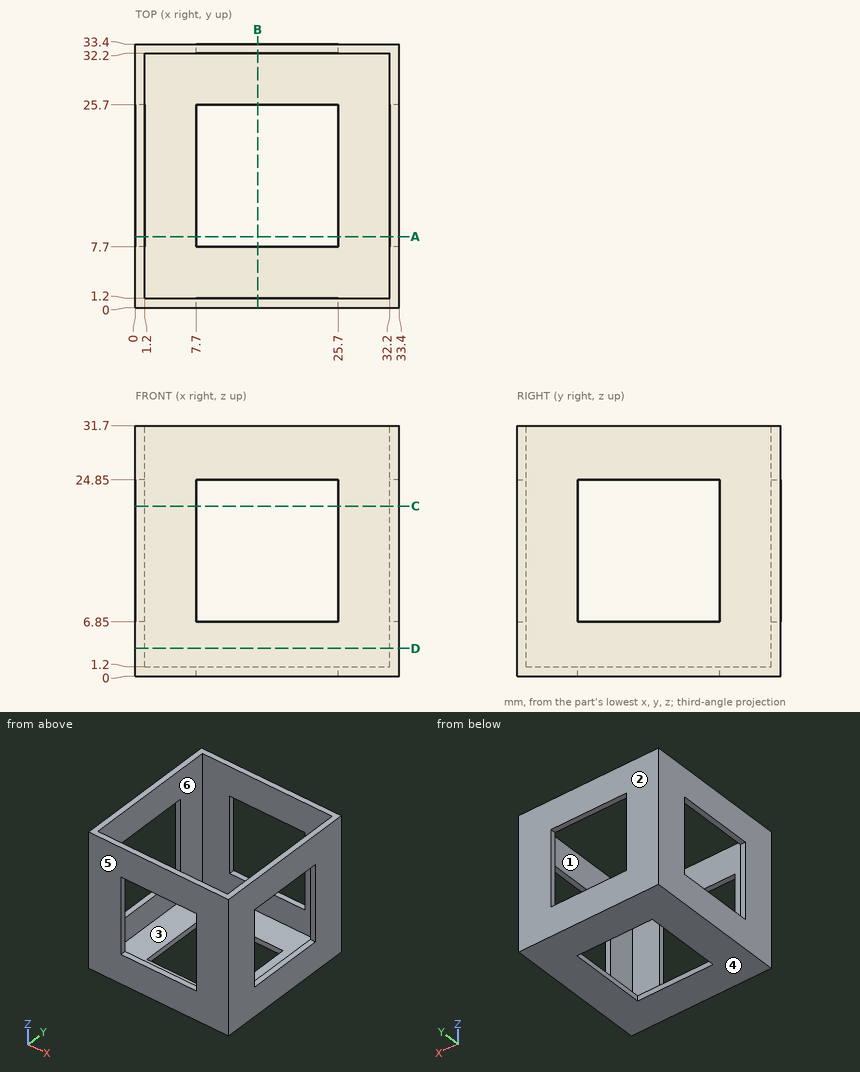
Design review of the part shown in the three views and the two pictorial views. Dimensions are in mm from the part's minimum x, y and z. A direction names the side the tool comes from. Round coordinates to 2 decimals unless told otherwise and drop trailing zeros. Order: outer loops, then holes, each group sorted by start corner. A loop starts at its lowest first (then second) coordinate and runs counter-clockwise, first axis right, second up. Notation, with made-up numbers: (-29, -23.5) -> (17, -23.5) arc R23 cw to (17, 12.5) -> close; hole circle Ø8 at (89, 31). An arc over 180 degrees is marked (long way). Write item = value, one per line. Start each with the question number.
1) Insertion check: pin 1 (3 mm diameter, centred on x = 15, z = 8, fed in from -Y); pin 2 (12 mm diameter, centred on x = 23.5, y = 21, fed in from +Z). Each pin has a flat end and moves straight along its axis. Give the tip position at first contact, or say it passes through.
2) Tool access review of the marked faces 5 and 6: name each direction out of +Z, -Z, +X, -X, +Y, -Y from which nothing blocks a thin tool from reaching the whole face with its end or side.
3) Take a section at A-A on y = 9. State the section outline as (x, z) points.
4) Take a section at D-D on z = 3.5. State the section outline as (x, y) points, plus the area to 3 significant figures.
5) To check wall thickness, follow line 1 (X direction, y = 15.5, z = 27); line 2 (Y direction, x = 18, z = 1). State the ranges of each line that lie inside material, in increasing order. Write a range as from..to.
6) Take a section at C-C on z = 21.5. State the section outline as (x, y) points, plus the area to 3 significant figures.
7) The part is to be moulded in two halves that separate along Y. For the marked faces 1, 2, 3 and 4, say which applies: +Y half, -Y half, draft (parallel to the pull), parting line (faces both ways), or undercut.
Verdict:
q1.pin_1 = 0
q1.pin_2 = 1.2
q2.face_5 = +Z, -Z, +X, -X, -Y
q2.face_6 = +Z
q3.outline = (0, 0) -> (7.7, 0) -> (7.7, 1.2) -> (1.2, 1.2) -> (1.2, 6.85) -> (0, 6.85) -> close; (0, 24.85) -> (1.2, 24.85) -> (1.2, 31.7) -> (0, 31.7) -> close; (25.7, 0) -> (33.4, 0) -> (33.4, 6.85) -> (32.2, 6.85) -> (32.2, 1.2) -> (25.7, 1.2) -> close; (32.2, 24.85) -> (33.4, 24.85) -> (33.4, 31.7) -> (32.2, 31.7) -> close
q4.outline = (0, 0) -> (33.4, 0) -> (33.4, 33.4) -> (0, 33.4) -> close; hole (1.2, 1.2) -> (32.2, 1.2) -> (32.2, 32.2) -> (1.2, 32.2) -> close
q4.area = 155 mm2
q5.line_1 = 0..1.2, 32.2..33.4
q5.line_2 = 0..7.7, 25.7..33.4
q6.outline = (0, 0) -> (7.7, 0) -> (7.7, 1.2) -> (1.2, 1.2) -> (1.2, 7.7) -> (0, 7.7) -> close; (0, 25.7) -> (1.2, 25.7) -> (1.2, 32.2) -> (7.7, 32.2) -> (7.7, 33.4) -> (0, 33.4) -> close; (25.7, 0) -> (33.4, 0) -> (33.4, 7.7) -> (32.2, 7.7) -> (32.2, 1.2) -> (25.7, 1.2) -> close; (25.7, 32.2) -> (32.2, 32.2) -> (32.2, 25.7) -> (33.4, 25.7) -> (33.4, 33.4) -> (25.7, 33.4) -> close
q6.area = 68.2 mm2
q7.face_1 = undercut
q7.face_2 = +Y half
q7.face_3 = undercut
q7.face_4 = draft
